Autodesk Inventor part; units mm, degrees
ref_plane "YZ Plane" through (0, 0, 0) normal (1, 0, 0) x (0, 1, 0)
ref_plane "XZ Plane" through (0, 0, 0) normal (0, 1, 0) x (-1, 0, 0)
ref_plane "XY Plane" through (0, 0, 0) normal (0, 0, 1) x (1, 0, 0)
sketch "Sketch1" plane through (0, 0, 0) normal (0, 1, 0) x (-1, 0, 0)
  line L0 (0, 0) -> (0, -287.501) construction
  line L1 (-3, 0) -> (-3, -287.501)
  line L2 (3, -287.501) -> (3, 0)
  arc A0 (3, 0) -> (-3, 0) centre (0, 0) ccw
  arc A1 (-3, -287.501) -> (3, -287.501) centre (0, -287.501) ccw
  circle A2 centre (0, 0) radius 1.5
  circle A3 centre (0, -287.501) radius 1.5
  circle A4 centre (0, -39.171) radius 1.5
  circle A5 centre (0, -94.738) radius 1.5
  circle A6 centre (0, -233.822) radius 1.5
  arc A7 (-3, -230.822) -> (-3, -97.738) centre (-800.2278, -164.28) ccw
  arc A8 (3, -230.822) -> (3, -97.738) centre (-794.2278, -164.28) ccw
  point P0 (0, -143.7505)
  dimension "d0" = 6
  dimension "d1" = 287.501
  dimension "d2" = 3
  dimension "d3" = 3
  dimension "d14" = 3
  dimension "d15" = 39.171
  dimension "d16" = 3
  dimension "d17" = 94.738
  dimension "d18" = 3
  dimension "d19" = 233.822
  dimension "d20" = 800
  dimension "d21" = 800
  dimension "d22" = 3
  dimension "d23" = 3
extrude "Extrusion1" add sketch "Sketch1" along normal blind 10 contours A0 L2 A1 L1 A7 | A8 L2
Here's how the part is built. I have some questions about the finished solid (model axes, mm). A direction names the side the tool comes from. Give positions to 0.01 mm unless a question says otherwise; leave off trailing zeros. Loops run counter-clockwise (first coordinate to the right, second up) from the corner with the lowest first, then second, coordinate; pieces in that order, holes last. Notation, with made-up numbers: M 75,-27 L 127,-27 A17 ccw 127,-11 Z; hole C 75.25,79.25 d8. An arc over 180 degrees is marked long. Put each result on its own line as item: value. Start each with the question number.
(1) I need wall thicknesses on line 1 along Z through (x, y) = (0, 4); line 2 along X through (y, z) = (6.75, -251.5); line 3 along Z through (x, y) = (-1.25, 2.75). Which ranges of each line are inside material? Lowest first, please. Write a range as [from, to].
(2) If we mould it in two halves opening along Z, with no side actions, what happens to faces 4 (the cylindrical face through (0.23, 4.93, -163.35)), 5 (the cylindrical face through (-5.77, 4.93, -163.35)), 6 (the flat face through (3, 5, -259))? For each: +Z half, -Z half, draft (parallel to the pull), parting line (faces both ways), or undercut.
(3) I want a section at A-A on y = 5.25. Please give me the cut outline in (x, z), then the cut area to 3 significant figures.
(4) Will these pins go through, and if not, where does the flat tip stop? pin 1 Ø3 at (x, y) = (-4, 6) entering from +Z; pin 2 Ø1 at (x, y) = (-1, 7.5) entering from +Z; pin 3 Ø3 at (x, y) = (-3, 6.5) entering from -Z; pin 4 Ø2.5 at (x, z) = (0, -39.171) entering from +Y.
(5) I want a section at B-B on z = -164. Please give me the cut outline in (x, y).
(6) For faces 1 (the flat face through (-3, 5, -260)), 2 (the cylindrical face through (0, 5, 3)), 3 (the flat face through (-3, 5, -50)), which set-ups out of +Z, -Z, +X, -X, +Y, -Y let a thin tool reach every point of the face, with its end or its side?
Answer block:
1. line 1: [-290.5, -289], [-286, -235.32], [-232.32, -96.24], [-93.24, -40.67], [-37.67, -1.5], [1.5, 3]
1. line 2: [-3, 3]
1. line 3: [-290.23, -288.33], [-286.67, -234.65], [-232.99, -95.57], [-93.91, -40], [-38.34, -0.83], [0.83, 2.73]
2. face 4: undercut
2. face 5: parting line
2. face 6: draft
3. outline: M -3,-287.5 A3 ccw 3,-287.5 L 3,-230.82 A800 cw 3,-97.74 L 3,0 A3 ccw -3,0 L -3,-97.74 A800 ccw -3,-230.82 Z; hole C 0,-287.5 d3; hole C 0,-233.82 d3; hole C 0,-94.74 d3; hole C 0,-39.17 d3; hole C 0,0 d3
3. area: 1,720 mm^2
4. pin 1: z = 1.66
4. pin 2: z = 2.96
4. pin 3: z = -290.1
4. pin 4: through
5. outline: M -5.77,0 L 0.23,0 L 0.23,10 L -5.77,10 Z
6. face 1: -Z, -X, +Y, -Y
6. face 2: +Z, +Y, -Y
6. face 3: +Z, -X, +Y, -Y
